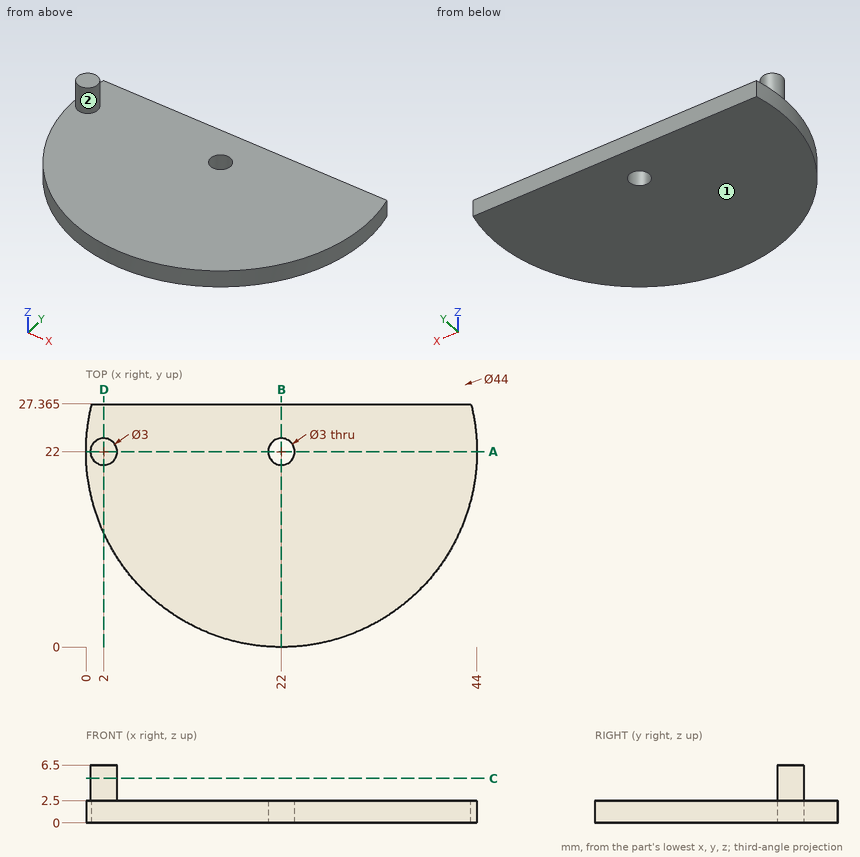
Verification items for this drawing (mm, ordinates from the low corner). Coordinates: 2 decimals unless noted, no trailing zeros. Loops run counter-clockwise (first coordinate to the right, second up) from the corner with the lowest first, then second, coordinate; pieces in that order, holes last. Notation, with made-up numbers: (33, -1) -> (72, -1) arc R33 ccw to (72, 34) -> close; hole circle Ø10 at (74.25, 67). An arc over 180 degrees is marked (long way). Answer in a Markdown table with one row per item. Add a question column.
1. Section check C-C, the plane z = 5. Enter the section's corners in (x, y).
2. Section check D-D, the plane x = 2. Enter the section's corners in (y, z) (1 decimal).
3. Section check A-A, the plane y = 22. Enter the section's corners in (x, z).
4. Depth check by flat-ended pin: P1, Ø13.5, axis at x = 20, y = 12, coming from the +Z side. Enter the tip coordinate at first touch or a pass-through.
5. Draft check along Y on the marked faces 1 and 2. Enter one of: +Y half, -Y half, draft (parallel to the pull), parting line (faces both ways), or undercut.
6. Section check B-B, the plane x = 22. Enter the section's corners in (y, z) (1 decimal).
7. Material ranges on probe 1 along Z at (x, y) = (39.5, 23.5); probe 2 along X at (y, z) = (17.75, 1.75) (1 decimal); probe 3 along X at (y, z) = (22.5, 3.5) (1 decimal), recorded low to high. Write a range as [from, to].
Derived:
| question | item | result |
|---|---|---|
| 1 | outline | circle Ø3 at (2, 22) |
| 2 | outline | (12.8, 0) -> (27.4, 0) -> (27.4, 2.5) -> (23.5, 2.5) -> (23.5, 6.5) -> (20.5, 6.5) -> (20.5, 2.5) -> (12.8, 2.5) -> close |
| 3 | outline | (0, 0) -> (20.5, 0) -> (20.5, 2.5) -> (3.5, 2.5) -> (3.5, 6.5) -> (0.5, 6.5) -> (0.5, 2.5) -> (0, 2.5) -> close; (23.5, 0) -> (44, 0) -> (44, 2.5) -> (23.5, 2.5) -> close |
| 4 | P1 | stops at z = 2.5 |
| 5 | face 1 | draft |
| 5 | face 2 | parting line |
| 6 | outline | (0, 0) -> (20.5, 0) -> (20.5, 2.5) -> (0, 2.5) -> close; (23.5, 0) -> (27.4, 0) -> (27.4, 2.5) -> (23.5, 2.5) -> close |
| 7 | probe 1 | z = [0, 2.5] |
| 7 | probe 2 | x = [0.4, 43.6] |
| 7 | probe 3 | x = [0.6, 3.4] |
